CAD build for the part. Positions are in the model's coordinates, mm. Face numbers are marked on the shaded views. Give positions to 0.01 mm unless a question says otherwise; leave off trailing zeros. Write each loop counter-clockwise with the first axis right and the second up, starting at its lowest first coordinate (ties: lowest second). Pieces come first, ordered by that corner, then holes. Notation, with made-up numbers: (-10, 9) - (3, 9) arc R25 ccw to (3, 39) - close; hole circle Ø1 at (66, 85). An arc over 180 degrees is marked (long way). Put each result on its own line as item: value. Start each with the question number.
1. Mould opens along Y. For the marked faces 1, 2 and 3 say: +Y half, -Y half, draft (parallel to the pull), parting line (faces both ways), or undercut.
2. Wall check: line 1 (Y direction, x = 0, z = 9.5); line 2 (Y direction, x = 0, z = 2); line 3 (Z direction, x = -0.75, y = 1.5). Give the ranges that are in metal, low to high.
3. Cut at C-C on z = 13. List the corners of the cut face in (x, y).
4. Cut at A-A on x = 0. List the corners of the cut face in (y, z), and give its area (3 significant figures).
5. Cut at D-D on z = 7.5. List the corners of the cut face in (x, y), and give its area (3 significant figures).
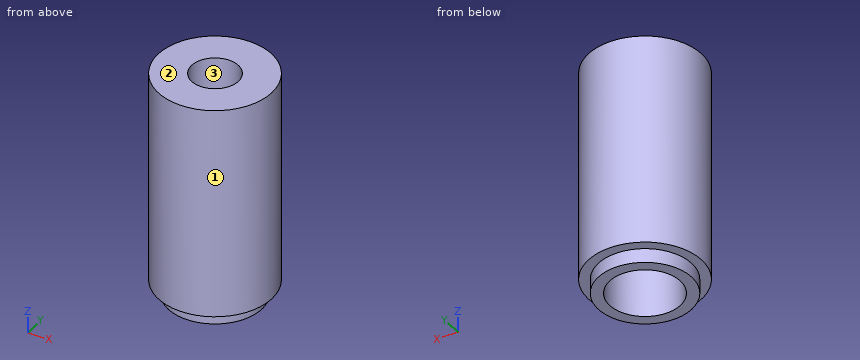
from build123d import *

# Parameters (mm, degrees)
ESQUISSE1_R             = 4
BOSS_EXTRU_1_DEPTH      = 16
TROU_TARAUD_M41_D       = 3.3
TROU_TARAUD_M41_DEPTH   = 8
TROU_TARAUD_M41_TIP     = 0.991420021
ESQUISSE4_R             = 2.5
ENL_V_MAT_EXTRU_1_DEPTH = 8
ESQUISSE5_OUTSIDE_W     = 13.92
ESQUISSE5_OUTSIDE_H     = 13.92
ESQUISSE5_OUTSIDE_R     = 3.3
ENL_V_MAT_EXTRU_2_DEPTH = 1


with BuildPart() as part:
    # Esquisse1 → Boss.-Extru.1 (new body)
    with BuildSketch(Plane.XY):
        Circle(ESQUISSE1_R)
    extrude(amount=BOSS_EXTRU_1_DEPTH)

    # Trou taraudé M41
    with Locations(Plane.XY.offset(16)):
        with Locations((0, 0)):
            Hole(TROU_TARAUD_M41_D / 2, depth=TROU_TARAUD_M41_DEPTH)
            with Locations((0, 0, -(TROU_TARAUD_M41_DEPTH + TROU_TARAUD_M41_TIP / 2))):  # 118° drill point
                Cone(0, TROU_TARAUD_M41_D / 2, TROU_TARAUD_M41_TIP, mode=Mode.SUBTRACT)

    # Esquisse4 → Enlèv. mat.-Extru.1 (cut)
    with BuildSketch(Plane(origin=(0, 0, 0), x_dir=(-1, 0, 0), z_dir=(0, 0, -1))):
        Circle(ESQUISSE4_R)
    extrude(amount=-ENL_V_MAT_EXTRU_1_DEPTH, mode=Mode.SUBTRACT)

    # Esquisse5 outside → Enlèv. mat.-Extru.2 (cut)
    with BuildSketch(Plane(origin=(0, 0, 0), x_dir=(-1, 0, 0), z_dir=(0, 0, -1))):
        Rectangle(ESQUISSE5_OUTSIDE_W, ESQUISSE5_OUTSIDE_H)
        Circle(ESQUISSE5_OUTSIDE_R, mode=Mode.SUBTRACT)
    extrude(amount=-ENL_V_MAT_EXTRU_2_DEPTH, mode=Mode.SUBTRACT)


solid = part.part
Report:
1. face 1: parting line
1. face 2: draft
1. face 3: undercut
2. line 1: y = -4 to -1.65, 1.65 to 4
2. line 2: y = -4 to -2.5, 2.5 to 4
2. line 3: z = 8 to 16
3. outline: circle Ø8 at (0, 0); hole circle Ø3.3 at (0, 0)
4. outline: (-4, 1) - (-3.3, 1) - (-3.3, 0) - (-2.5, 0) - (-2.5, 8) - (-1.65, 8) - (-1.65, 16) - (-4, 16) - close; (1.65, 8) - (2.5, 8) - (2.5, 0) - (3.3, 0) - (3.3, 1) - (4, 1) - (4, 16) - (1.65, 16) - close
4. area: 60.2 mm²
5. outline: circle Ø8 at (0, 0); hole circle Ø5 at (0, 0)
5. area: 30.6 mm²
